from build123d import *

# Parameters (mm, degrees)
SKETCH3_W                = 4
SKETCH3_H                = 73.62
BOSS_EXTRUDE2_DEPTH      = 110
BOSS_EXTRUDE2_2_DEPTH    = 110
SKETCH4_OUTSIDE_W        = 140.16
SKETCH4_OUTSIDE_H        = 103.78
CUT_EXTRUDE1_DEPTH       = 110
BOSS_EXTRUDE3_DEPTH      = 40
SKETCH6_R                = 7
SKETCH6_R_2              = 6
CUT_EXTRUDE2_DEPTH       = 110
SKETCH7_R                = 37
SKETCH7_R_2              = 26
BOSS_EXTRUDE4_DEPTH      = 73.7
BOSS_EXTRUDE6_START      = -73.7
BOSS_EXTRUDE6_DEPTH      = 73.7
CUT_EXTRUDE9_START       = -60
CUT_EXTRUDE9_DEPTH       = 60
SKETCH15_R               = 10
CUT_EXTRUDE11_DEPTH      = 74
BOSS_EXTRUDE8_REACH      = 171.943
CUT_EXTRUDE12_DEPTH      = 172.60636515
CUT_EXTRUDE12_DEPTH_BACK = 172.60636515
SKETCH18_W               = 0.383748065
SKETCH18_H               = 73.7
BOSS_EXTRUDE9_START      = -5
BOSS_EXTRUDE9_DEPTH      = 5
CUT_EXTRUDE13_DEPTH      = 50


# Read off the part's stored shape, not the designer's step: Cut-Extrude9
with BuildPart() as part:
    # Sketch3 → Boss-Extrude2 (new body)
    with BuildSketch(Plane.XY):
        with Locations((2, 36.81)):
            Rectangle(SKETCH3_W, SKETCH3_H)
    extrude(amount=BOSS_EXTRUDE2_DEPTH)


with BuildPart() as body_2:
    # Sketch3 → Boss-Extrude2 2 (new body)
    with BuildSketch(Plane.XY):
        with Locations((46, 36.81)):
            Rectangle(SKETCH3_W, SKETCH3_H)
    extrude(amount=BOSS_EXTRUDE2_2_DEPTH)


with BuildPart() as cut_extrude1_tool:
    # Sketch4 outside → Cut-Extrude1 (new body)
    with BuildSketch(Plane(origin=(48, 0, 0), x_dir=(0, 0, -1), z_dir=(1, 0, 0))):
        with Locations((-55, 36.81)):
            Rectangle(SKETCH4_OUTSIDE_W, SKETCH4_OUTSIDE_H)
        with BuildLine():
            Line((0, 5.709271206), (-99.676636629, -0.093636173))
            add(Edge.make_bspline(
                [(-96.468976077, 19.025739265), (-149.450115124, -2.991315062), (-99.676636629, -0.093636173)],
                knots=[1.570796327, 1.570796327, 1.570796327, 4.103862701, 4.103862701, 4.103862701], degree=2, weights=[1, 0.299590242, 1]))
            Line((-96.468976077, 19.025739265), (0, 73.62))
            Line((0, 73.62), (0, 5.709271206))
        make_face(mode=Mode.SUBTRACT)
    extrude(amount=-CUT_EXTRUDE1_DEPTH)


with BuildPart() as part_1:
    add(part.part)

    # Cut-Extrude1: cut by cut_extrude1_tool
    add(cut_extrude1_tool.part, mode=Mode.SUBTRACT)



with BuildPart() as body_2_1:
    add(body_2.part)

    # Cut-Extrude1: cut by cut_extrude1_tool
    add(cut_extrude1_tool.part, mode=Mode.SUBTRACT)


with BuildPart() as part_2:
    add(part_1.part)

    add(body_2_1.part)  # Boss-Extrude3 merges body 2
    # Sketch5 → Boss-Extrude3 (add)
    with BuildSketch(Plane(origin=(4, 0, 0), x_dir=(0, 0, -1), z_dir=(1, 0, 0))):
        Polygon((0, 73.62), (-85.221110514, 25.391194049), (-83.506537519, 22.361514757), (0, 69.62), align=None)
    extrude(amount=BOSS_EXTRUDE3_DEPTH)

    # Sketch6 → Cut-Extrude2 (cut)
    with BuildSketch(Plane(origin=(48, 0, 0), x_dir=(0, 0, -1), z_dir=(1, 0, 0))):
        with Locations(Location((-43.596276135, 22.110704559, 0), (0, 0, 90))):
            Circle(SKETCH6_R)
        with Locations(Location((-85.5494254, 13.322513691, 0), (0, 0, 90))):
            Circle(SKETCH6_R_2)
    extrude(amount=-CUT_EXTRUDE2_DEPTH, mode=Mode.SUBTRACT)

    # Sketch7 → Boss-Extrude4 (add)
    with BuildSketch(Plane(origin=(0, 0, 0), x_dir=(1, 0, 0), z_dir=(0, 1, 0))):
        with Locations(Location((24, 28.160255681, 0), (0, 0, 270))):
            Circle(SKETCH7_R)
        with Locations(Location((24, 28.160255681, 0), (0, 0, 270))):
            Circle(SKETCH7_R_2, mode=Mode.SUBTRACT)
    extrude(amount=BOSS_EXTRUDE4_DEPTH)

    # Sketch9 → Boss-Extrude6 (add)
    with BuildSketch(Plane(origin=(0, 73.7, 0), x_dir=(1, 0, 0), z_dir=(0, 1, 0)).offset(BOSS_EXTRUDE6_START)):
        with BuildLine():
            ThreePointArc((56, 46.734431302), (58.367878709, 41.866054199), (60, 36.704259426))
            Line((60, 36.704259426), (60, 136.704259426))
            Line((60, 136.704259426), (56, 136.704259426))
            Line((56, 136.704259426), (56, 46.734431302))
        make_face()
        with BuildLine():
            Line((0, 136.320511361), (0, 56.320511361))
            ThreePointArc((0, 56.320511361), (1.949988398, 57.872155458), (4, 59.289020513))
            Line((4, 59.289020513), (4, 136.320511361))
            Line((4, 136.320511361), (0, 136.320511361))
        make_face()
    extrude(amount=BOSS_EXTRUDE6_DEPTH)

    # Cut-Extrude9 outline → Cut-Extrude9 (cut)
    with BuildSketch(Plane.ZY.offset(CUT_EXTRUDE9_START)):
        with BuildLine():
            add(Edge.make_bspline(
                [(-136.320511361, 36.85), (-136.320511361, 27.575850811), (-117.029991726, 20.926444667)],
                knots=[6.283185307, 6.283185307, 6.283185307, 7.054517173, 7.054517173, 7.054517173], degree=2, weights=[0.858491437, 0.858491437, 1]))
            Line((-136.320511361, 36.85), (-136.320511361, 0))
            Line((-136.320511361, 0), (-56.320511361, 0))
            Line((-56.320511361, 0), (-117.029991726, 20.926444667))
        make_face()
        with BuildLine():
            add(Edge.make_bspline(
                [(-117.029991726, 52.773555333), (-136.320511361, 46.124149189), (-136.320511361, 36.85)],
                knots=[5.511853442, 5.511853442, 5.511853442, 6.283185307, 6.283185307, 6.283185307], degree=2, weights=[1, 0.858491437, 0.858491437]))
            Line((-117.029991726, 52.773555333), (-56.320511361, 73.7))
            Line((-56.320511361, 73.7), (-136.320511361, 73.7))
            Line((-136.320511361, 73.7), (-136.320511361, 36.85))
        make_face()
    extrude(amount=CUT_EXTRUDE9_DEPTH, mode=Mode.SUBTRACT)

    # Sketch15 → Cut-Extrude11 (cut)
    with BuildSketch(Plane(origin=(60, 0, 0), x_dir=(0, 0, -1), z_dir=(1, 0, 0))):
        with Locations((103.144942626, 35.814780524)):
            Circle(SKETCH15_R)
    extrude(amount=-CUT_EXTRUDE11_DEPTH, mode=Mode.SUBTRACT)

    # Boss-Extrude8: up to this face of the body (flat: up to its plane)
    boss_extrude8_end = Plane(part_2.part.faces().sort_by_distance((4, 36.955026581, -88.076596364))[0])
    # Sketch16 → Boss-Extrude8 (add, up to the picked face)
    with BuildSketch(Plane.ZY.offset(-56), mode=Mode.PRIVATE) as boss_extrude8_sk1:
        Polygon((-58.244155034, 73.036923613), (-81.124851518, 65.149990205), (-79.821326308, 61.368347436), (-58.244155034, 68.805958136), align=None)
    boss_extrude8_tool1 = split(extrude(boss_extrude8_sk1.sketch, amount=BOSS_EXTRUDE8_REACH, mode=Mode.PRIVATE), bisect_by=boss_extrude8_end, keep=Keep.BOTH, mode=Mode.PRIVATE)
    add(boss_extrude8_tool1.solids().sort_by(Axis((56, 67.109883, -69.361807), (-1, 0, 0)))[0])

    # Sketch18 → Cut-Extrude12 (cut, two sides: drawn at the far end of the back side and taken through both)
    with BuildSketch(Plane(origin=(60, 0, 0), x_dir=(0, 0, -1), z_dir=(1, 0, 0)).offset(-CUT_EXTRUDE12_DEPTH_BACK)):
        with Locations((136.512385394, 36.85)):
            Rectangle(SKETCH18_W, SKETCH18_H)
    extrude(amount=CUT_EXTRUDE12_DEPTH + CUT_EXTRUDE12_DEPTH_BACK, mode=Mode.SUBTRACT)

    # Sketch19 → Boss-Extrude9 (add)
    with BuildSketch(Plane(origin=(0, 73.7, 0), x_dir=(1, 0, 0), z_dir=(0, 1, 0)).offset(BOSS_EXTRUDE9_START)):
        with BuildLine():
            Line((56, 56.320511361), (56, 58.244155034))
            Line((56, 58.244155034), (45.539707511, 58.244155034))
            ThreePointArc((45.539707511, 58.244155034), (46.79015887, 57.308302934), (48, 56.320511361))
            ThreePointArc((48, 56.320511361), (52.407274292, 51.867359411), (56, 46.734431302))
            Line((56, 46.734431302), (56, 56.320511361))
        make_face()
    extrude(amount=BOSS_EXTRUDE9_DEPTH)

    # Sketch20 → Cut-Extrude13 (cut)
    with BuildSketch(Plane(origin=(60, 0, 0), x_dir=(0, 0, -1), z_dir=(1, 0, 0))):
        Polygon((58.244155034, 73.036923613), (58.244155034, 73.7), (56.320511361, 73.7), align=None)
    extrude(amount=-CUT_EXTRUDE13_DEPTH, mode=Mode.SUBTRACT)


solid = part_2.part
Check sheet for the modelled part. Datum: model origin and axes. Units: mm. A direction names the side the tool comes from. Coordinates: 2 decimals unless noted, no trailing zeros. Write each loop counter-clockwise with the first axis right and the second up, starting at its lowest first coordinate (ties: lowest second). Pieces come first, ordered by that corner, then holes.
Item 1: Cross-section at C-C on z = -11. Record the boundary of the cut face in (x, y).
Numbers:
outline: (-8.78, 0) - (4.47, 0) - (4.47, 73.7) - (-8.78, 73.7) - close; (43.53, 0) - (56.78, 0) - (56.78, 73.7) - (43.53, 73.7) - close
Item 2: Cross-section at B-B on x = 15.5. Record the boundary of the cut face in (y, z).
Numbers:
outline: (0, -56.32) - (2.71, -64.17) - (66.76, -64.17) - (61.37, -79.82) - (65.15, -81.12) - (73.7, -56.32) - (73.7, -52.73) - (0, -52.73) - close; (0, -3.59) - (73.7, -3.59) - (73.7, 7.85) - (69.18, 7.85) - (25.39, 85.22) - (22.36, 83.51) - (65.18, 7.85) - (0, 7.85) - close
Item 3: Cross-section at D-D on y = 32. Count the separate pieces of the cut face and the enclosed holes in it, then the cut area to 3 significant figures.
Numbers:
separate pieces: 3
enclosed holes: 2
area: 3,560 mm2
Item 4: Cross-section at A-A on z = -44.5. Record the boundary of the cut face in (x, y).
Numbers:
outline: (-9.2, 0) - (3.78, 0) - (3.78, 73.7) - (-9.2, 73.7) - close; (44.22, 0) - (60, 0) - (60, 73.7) - (44.22, 73.7) - close
Item 5: Depth check by flat-ended pin: pin 1 Ø12.5 at (y, z) = (22.11, 43.6) entering from -X; pin 2 Ø3 at (x, z) = (30, 80) entering from -Y; pin 3 Ø1 at (x, y) = (30, 26.5) entering from +Z; pin 4 Ø2 at (x, y) = (13.5, 45) entering from -Z. Enter the tip coordinate at first touch or a pass-through.
Numbers:
pin 1: passes through
pin 2: stops at y = 23.5
pin 3: stops at z = 84.15
pin 4: stops at z = -63.92
Item 6: Mould release check, pull along Y, two halves, no side actions. Record for faces 4 (the face through (33, 73.7, -2)), 5 (the face through (58.028, 44.247, -108.521)), 6 (the face through (46.028, 2.895, 48.348)): released by +Y, released by -Y, zero draft, split by the parting line, or undercut.
Numbers:
face 4: released by +Y
face 5: undercut
face 6: released by -Y
Item 7: Access from +Z, -Z, +X, -X, +Y, -Y to the whole of each face (thin tool, end or side, straight path). Record for faces 1 (the face through (44, 33, 44)), 2 (the face through (48, 36, 42)), 3 (the face through (60, 36, -75)).
Numbers:
face 1: -Y
face 2: +Z, +X, +Y, -Y
face 3: -Z, +X, +Y, -Y
Item 8: Scan lines: probe 1 along X at (y, z) = (13, 53); probe 2 along Z at (x, y) = (12, 48); probe 3 along X at (y, z) = (36, -123). Record each from-to range of solid material in increasing order.
Numbers:
probe 1: x = 0 to 4, 44 to 48
probe 2: z = -63.16 to -51.23, -5.1 to 6.84, 38.2 to 45.27
probe 3: x = 0 to 4, 56 to 60
